```python
from build123d import *

# Parameters (mm, degrees)
SKETCH1_R                    = 4.7625
BOSS_EXTRUDE1_DEPTH          = 25.4
SKETCH2_R                    = 3.9751
BOSS_EXTRUDE2_DEPTH          = 7.366
SKETCH3_R                    = 3.0226
CUT_EXTRUDE1_DEPTH           = 33.766
F_5_16_24_TAPPED_HOLE1_D     = 6.9088
F_5_16_24_TAPPED_HOLE1_DEPTH = 12.7
F_5_16_24_TAPPED_HOLE1_TIP   = 2.075612922


with BuildPart() as part:
    # Sketch1 → Boss-Extrude1 (new body)
    with BuildSketch(Plane(origin=(0, 0, 0), x_dir=(1, 0, 0), z_dir=(0, 1, 0))):
        with Locations(Location((0, 0, 0), (0, 0, 270))):  # turned: the seam where the file's is
            Circle(SKETCH1_R)
    extrude(amount=BOSS_EXTRUDE1_DEPTH)

    # Sketch2 → Boss-Extrude2 (add)
    with BuildSketch(Plane(origin=(0, 25.4, 0), x_dir=(1, 0, 0), z_dir=(0, 1, 0))):
        with Locations(Location((0, 0, 0), (0, 0, 270))):  # turned: the seam where the file's is
            Circle(SKETCH2_R)
    extrude(amount=BOSS_EXTRUDE2_DEPTH)

    # Sketch3 → Cut-Extrude1 (cut, through all)
    with BuildSketch(Plane.XZ):
        with Locations(Location((0, 0, 0), (0, 0, 270))):  # turned: the seam where the file's is
            Circle(SKETCH3_R)
    extrude(amount=-CUT_EXTRUDE1_DEPTH, mode=Mode.SUBTRACT)

    # 5/16-24 Tapped Hole1
    with Locations(Plane(origin=(0, 0, 0), x_dir=(-1, 0, 0), z_dir=(0, -1, 0))):
        with Locations((0, 0)):
            Hole(F_5_16_24_TAPPED_HOLE1_D / 2, depth=F_5_16_24_TAPPED_HOLE1_DEPTH)
            with Locations((0, 0, -(F_5_16_24_TAPPED_HOLE1_DEPTH + F_5_16_24_TAPPED_HOLE1_TIP / 2))):  # 118° drill point
                Cone(0, F_5_16_24_TAPPED_HOLE1_D / 2, F_5_16_24_TAPPED_HOLE1_TIP, mode=Mode.SUBTRACT)


solid = part.part
```
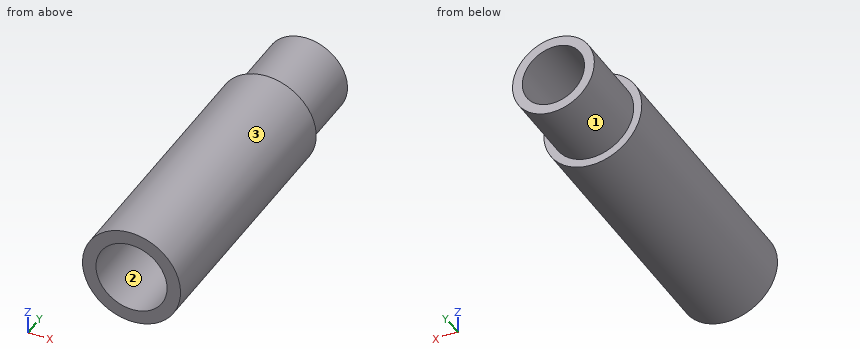
Build history of the part. All positions in model axes, mm. Face numbers are marked on the shaded views. A direction names the side the tool comes from. Round coordinates to 2 decimals unless told otherwise and drop trailing zeros. Order: outer loops, then holes, each group sorted by start corner. A loop starts at its lowest first (then second) coordinate and runs counter-clockwise, first axis right, second up. Notation, with made-up numbers: (-15, -17.75) - (15, -17.75) arc R11 ccw to (15, -5.75) - close; hole circle Ø2 at (-32, -11.5). An arc over 180 degrees is marked (long way). Use a Markdown table: item, result.
1) Saw through at D-D on y = 28.5. Write the cut outline in (x, z), and give its area (3 significant figures).
Recorded:
| item | result |
|---|---|
| outline | circle Ø7.95 at (0, 0); hole circle Ø6.05 at (0, 0) |
| area | 20.9 mm² |
2) Saw through at B-B on z = 0. Write the cut outline in (x, y).
Recorded:
| item | result |
|---|---|
| outline | (-4.76, 0) - (-3.45, 0) - (-3.45, 12.7) - (-3.02, 12.96) - (-3.02, 32.77) - (-3.98, 32.77) - (-3.98, 25.4) - (-4.76, 25.4) - close; (3.02, 12.96) - (3.45, 12.7) - (3.45, 0) - (4.76, 0) - (4.76, 25.4) - (3.98, 25.4) - (3.98, 32.77) - (3.02, 32.77) - close |
3) Saw through at A-A on x = 0. Write the cut outline in (y, z).
Recorded:
| item | result |
|---|---|
| outline | (0, -4.76) - (25.4, -4.76) - (25.4, -3.98) - (32.77, -3.98) - (32.77, -3.02) - (12.96, -3.02) - (12.7, -3.45) - (0, -3.45) - close; (0, 3.45) - (12.7, 3.45) - (12.96, 3.02) - (32.77, 3.02) - (32.77, 3.98) - (25.4, 3.98) - (25.4, 4.76) - (0, 4.76) - close |
4) Tool access for the marked faces 1, 2 and 3: list every direction of +Z, -Z, +X, -X, +Y, -Y with a clear straight run to the whole face (end or side of a thin tool).
Recorded:
| item | result |
|---|---|
| face 1 | +Y |
| face 2 | -Y |
| face 3 | +Y, -Y |
5) Wall check: L1, parallel to X at y = 31, z = 0; L2, parallel to X at y = 19.75, z = 0; L3, parallel to Z at x = 0.5, y = 12. Give the ranges that are in metal, low to high.
Recorded:
| item | result |
|---|---|
| L1 | x = -3.98 to -3.02, 3.02 to 3.98 |
| L2 | x = -4.76 to -3.02, 3.02 to 4.76 |
| L3 | z = -4.74 to -3.42, 3.42 to 4.74 |
6) Saw through at C-C on y = 16. Write the cut outline in (x, z) (1 decimal).
Recorded:
| item | result |
|---|---|
| outline | circle Ø9.5 at (0, 0); hole circle Ø6 at (0, 0) |
7) Flat gauge pins, fed straight in: pin 1 Ø3.5 at (x, z) = (0, 0) entering from +Y (3 decimals); pin 2 Ø5 at (x, y) = (-3, 16) entering from +Z. Where does each tip first touch, or does it go through?
Recorded:
| item | result |
|---|---|
| pin 1 | passes through |
| pin 2 | stops at z = 4.74 |
